Geometry check sheet. Reference: the model listing, model coordinates, mm. A direction names the side the tool comes from. Give positions to 0.01 mm unless a question says otherwise; leave off trailing zeros. Loops run counter-clockwise (first coordinate to the right, second up) from the corner with the lowest first, then second, coordinate; pieces in that order, holes last. Notation, with made-up numbers: (-0.75, -13) -> (13.25, -13) arc R20 cw to (13.25, 20) -> close; hole circle Ø11 at (49, -18). An arc over 180 degrees is marked (long way). One line per question, with ' | ' between items.
from build123d import *

# Parameters (mm, degrees)
SKETCH_2_W          = 12
SKETCH_2_H          = 9
EXTRUDE_1_DEPTH     = 80
SKETCH_3_R          = 3
CUT_EXTRUDE_1_DEPTH = 15
SKETCH_4_R          = 2.5
CUT_EXTRUDE_2_DEPTH = 15


with BuildPart() as part:
    # 草图2 → 凸台-拉伸1 (new body)
    with BuildSketch(Plane(origin=(0, 0, 0), x_dir=(1, 0, 0), z_dir=(0, 1, 0))):
        Rectangle(SKETCH_2_W, SKETCH_2_H)
    extrude(amount=EXTRUDE_1_DEPTH)

    # 草图3 → 切除-拉伸1 (cut)
    with BuildSketch(Plane.XZ):
        with Locations(Location((0, 0, 0), (0, 0, 270))):
            Circle(SKETCH_3_R)
    extrude(amount=-CUT_EXTRUDE_1_DEPTH, mode=Mode.SUBTRACT)

    # 草图4 → 切除-拉伸2 (cut)
    with BuildSketch(Plane(origin=(0, 80, 0), x_dir=(1, 0, 0), z_dir=(0, 1, 0))):
        with Locations(Location((0, 0, 0), (0, 0, 270))):
            Circle(SKETCH_4_R)
    extrude(amount=-CUT_EXTRUDE_2_DEPTH, mode=Mode.SUBTRACT)


solid = part.part
Item 1: Sectioned sample at B-B (z = 0). Record the cut outline in (x, y), plus the area to 3 significant figures.
Result:
outline: (-6, 0) -> (-3, 0) -> (-3, 15) -> (3, 15) -> (3, 0) -> (6, 0) -> (6, 80) -> (2.5, 80) -> (2.5, 65) -> (-2.5, 65) -> (-2.5, 80) -> (-6, 80) -> close | area: 795 mm2
Item 2: Sectioned sample at A-A (x = 0). Record the cut outline in (y, z), plus the area to 3 significant figures.
Result:
outline: (0, -4.5) -> (80, -4.5) -> (80, -2.5) -> (65, -2.5) -> (65, 2.5) -> (80, 2.5) -> (80, 4.5) -> (0, 4.5) -> (0, 3) -> (15, 3) -> (15, -3) -> (0, -3) -> close | area: 555 mm2
Item 3: Set-up check for faces 4 (the face through (-1, 0, -3)), 5 (the face through (0.9, 7.4, -2.86)), 6 (the face through (0, 65, 0)): record each of +Z, -Z, +X, -X, +Y, -Y from which the full face is reachable in a straight line by a thin tool's end or side.
Result:
face 4: +Z, -Z, +X, -X, -Y | face 5: -Y | face 6: +Y
Item 4: Scan lines: probe 1 along X at (y, z) = (12, 0); probe 2 along X at (y, z) = (71, 0); probe 3 along Y at (x, z) = (0.5, -2.5). Record each from-to range of solid material in increasing order.
Result:
probe 1: -6 to -3, 3 to 6 | probe 2: -6 to -2.5, 2.5 to 6 | probe 3: 15 to 80
Item 5: Depth check by flat-ended pin: pin 1 Ø3 at (x, z) = (0, 0) entering from +Y. Enter the tip coordinate at first touch or a pass-through.
Result:
pin 1: y = 65
Item 6: Release check for a two-part mould opening along Z. For faces 1 (the face through (0, 39, -4.5)), 2 (the face through (0, 15, 0)), 3 (the face through (6, 39, 0)) record: pulls with the +Z half, pulls with the -Z half, needs draft (parallel to the pull), parting line crosses it, or undercut.
Result:
face 1: pulls with the -Z half | face 2: undercut | face 3: needs draft
